from build123d import *

# Parameters (mm, degrees)
SKETCH1_R           = 69.85
BOSS_EXTRUDE1_DEPTH = 3.81
SKETCH2_R           = 63.5
SKETCH2_R_2         = 57.2897
BOSS_EXTRUDE2_DEPTH = 10.16
SKETCH3_R           = 50.546
SKETCH3_R_2         = 48.006
BOSS_EXTRUDE3_DEPTH = 10.16


with BuildPart() as part:
    # Sketch1 → Boss-Extrude1 (new body)
    with BuildSketch(Plane(origin=(0, 0, 0), x_dir=(1, 0, 0), z_dir=(0, 1, 0))):
        with Locations(Location((0, 0, 0), (0, 0, 90))):
            Circle(SKETCH1_R)
    extrude(amount=BOSS_EXTRUDE1_DEPTH)

    # Sketch2 → Boss-Extrude2 (add)
    with BuildSketch(Plane(origin=(0, 3.81, 0), x_dir=(1, 0, 0), z_dir=(0, 1, 0))):
        with Locations(Location((0, 0, 0), (0, 0, 270))):
            Circle(SKETCH2_R)
        with Locations(Location((0, 0, 0), (0, 0, 270))):
            Circle(SKETCH2_R_2, mode=Mode.SUBTRACT)
    extrude(amount=BOSS_EXTRUDE2_DEPTH)

    # Sketch3 → Boss-Extrude3 (add)
    with BuildSketch(Plane(origin=(0, 3.81, 0), x_dir=(1, 0, 0), z_dir=(0, 1, 0))):
        with Locations(Location((0, 0, 0), (0, 0, 270))):
            Circle(SKETCH3_R)
        with Locations(Location((0, 0, 0), (0, 0, 270))):
            Circle(SKETCH3_R_2, mode=Mode.SUBTRACT)
    extrude(amount=BOSS_EXTRUDE3_DEPTH)

    # Loft1: read off the stored shape, not the designer's step
    # Loft1: loft between two sections, ruled curve by curve
    loft1_from = [
        Edge.make_bspline([(-1.815697125, 9.652, 0.82394245), (-3.463582025, 9.652, -2.8074518), (0.167812225, 9.652, -4.4553367), (1.815697125, 9.652, -0.82394245), (3.463582025, 9.652, 2.8074518), (-0.167812225, 9.652, 4.4553367), (-1.815697125, 9.652, 0.82394245)], [0, 0, 0, 0, 0.5, 0.5, 0.5, 1, 1, 1, 1], 3, [1, 0.333333333, 0.333333333, 1, 0.333333333, 0.333333333, 1]),
    ]
    loft1_to = [
        Edge.make_bspline([(4.253244453, 3.81, 14.369763659), (-24.486282866, 3.81, 22.876252565), (-32.992771771, 3.81, -5.863274754), (-4.253244453, 3.81, -14.369763659), (24.486282866, 3.81, -22.876252565), (32.992771771, 3.81, 5.863274754), (4.253244453, 3.81, 14.369763659)], [0, 0, 0, 0, 0.5, 0.5, 0.5, 1, 1, 1, 1], 3, [1, 0.333333333, 0.333333333, 1, 0.333333333, 0.333333333, 1]),
    ]
    loft1 = Solid(Shell([*[Face.make_surface_from_curves(loft1_from[k], loft1_to[k]) for k in range(1)], Face(Wire(loft1_from)), Face(Wire(loft1_to))]))
    add(loft1)


solid = part.part
The model under review builds one solid part; all positions refer to its coordinate system, in mm. A direction names the side the tool comes from. Round coordinates to 2 decimals unless told otherwise and drop trailing zeros. Write each loop counter-clockwise with the first axis right and the second up, starting at its lowest first coordinate (ties: lowest second). Pieces come first, ordered by that corner, then holes. Notation, with made-up numbers: (69.5, 53) - (114.5, 53) arc R30 cw to (114.5, 85) - close; hole circle Ø7 at (0.5, 79.5). An arc over 180 degrees is marked (long way). One line per item, written item: value. Start each with the question number.
1. The part is to be moulded in two halves that separate along X. For faces 1 (the face through (57, 13.97, -10)), 2 (the face through (-46.864, 8.819, -10.407)), 3 (the face through (-61.99, 8.82, -13.77)), say which applies: released by +X, released by -X, zero draft, split by the parting line, or undercut.
2. Machinability: for faces 4 (the face through (68.2, 1.9, 15.1)), 5 (the face through (62, 3.81, -15)), which of the approach directions +Z, -Z, +X, -X, +Y, -Y give a long, thin tool a straight path to every point of the face, cutting with its end or side? Answer none if there is none.
3. Consider section C-C on y = 7. State how many separate pieces and enclosed holes the cut face has, and give its area (3 significant figures).
4. Consider section B-B on z = -17. Write out the cut boundary in (x, y), and give its area (3 significant figures).
5. To check wall thickness, follow L1, parallel to X at y = 9.75, z = 0; L2, parallel to Z at x = -28, y = 9.75; L3, parallel to X at y = 9.25, z = 42. State the ranges of each line that lie inside material, in increasing order. Write a range as from..to.
6. Clearance check with flat-ended pins moving along their axes: P1, Ø4.5, axis at x = 0, z = -1, coming from the +Y side; P2, Ø1.5, axis at y = 10.5, z = 49, coming from the +X side; P3, Ø1.5, axis at x = 25, z = -17, coming from the +Y side. State where each tip first meets the part, or that it passes through.
7. Consider section A-A on x = -45. Write out the cut boundary in (y, z), and give its area (3 significant figures).
Checks:
1. face 1: zero draft
1. face 2: undercut
1. face 3: split by the parting line
2. face 4: +Y, -Y
2. face 5: +Y
3. separate pieces: 3
3. enclosed holes: 2
3. area: 3,300 mm^2
4. outline: (-67.75, 0) - (67.75, 0) - (67.75, 3.81) - (61.18, 3.81) - (61.18, 13.97) - (54.71, 13.97) - (54.71, 3.81) - (47.6, 3.81) - (47.6, 13.97) - (44.9, 13.97) - (44.9, 3.81) - (-44.9, 3.81) - (-44.9, 13.97) - (-47.6, 13.97) - (-47.6, 3.81) - (-54.71, 3.81) - (-54.71, 13.97) - (-61.18, 13.97) - (-61.18, 3.81) - (-67.75, 3.81) - close
4. area: 703 mm^2
5. L1: x = -63.5..-57.29, -50.55..-48.01, 48.01..50.55, 57.29..63.5
5. L2: z = -56.99..-49.98, -42.08..-38.99, 38.99..42.08, 49.98..56.99
5. L3: x = -47.63..-38.96, -28.12..-23.25, 23.25..28.12, 38.96..47.63
6. P1: stops at y = 9.65
6. P2: stops at x = 41.28
6. P3: stops at y = 3.81
7. outline: (0, -53.42) - (3.81, -53.42) - (3.81, -44.8) - (13.97, -44.8) - (13.97, -35.46) - (3.81, -35.46) - (3.81, -23.02) - (13.97, -23.02) - (13.97, -16.72) - (3.81, -16.72) - (3.81, 16.72) - (13.97, 16.72) - (13.97, 23.02) - (3.81, 23.02) - (3.81, 35.46) - (13.97, 35.46) - (13.97, 44.8) - (3.81, 44.8) - (3.81, 53.42) - (0, 53.42) - close
7. area: 725 mm^2
